The model under review builds one solid part; all positions refer to its coordinate system, in mm. Face numbers are marked on the shaded views. A direction names the side the tool comes from. Round coordinates to 2 decimals unless told otherwise and drop trailing zeros. Loops run counter-clockwise (first coordinate to the right, second up) from the corner with the lowest first, then second, coordinate; pieces in that order, holes last. Notation, with made-up numbers: (-31.5, 20.5) -> (8.5, 20.5) arc R23 cw to (8.5, 44.5) -> close; hole circle Ø10 at (88.25, 5.5). An arc over 180 degrees is marked (long way). Return JSON: item names as keys, results as strings. Group by question number.
```python
from build123d import *

# Parameters (mm, degrees)
F0_W          = 24
F0_H          = 25
F1_DEPTH      = 2
F2_R          = 6.25
F3_DEPTH      = 3
F4_W          = 24
F4_H          = 2
F5_DEPTH      = 7
F5_DEPTH_BACK = 2
F7_START      = 12
F6_W          = 4.5
F6_H          = 5
F7_DEPTH      = 3
F8_START      = -12
F8_DEPTH      = 3
F9_R          = 0.5


with BuildPart() as f1:
    # F0 (on Top) → F1 (new body)
    with BuildSketch(Plane.XY):
        Rectangle(F0_W, F0_H)
    extrude(amount=-F1_DEPTH)

    # F2 (on Top) → F3 (join)
    with BuildSketch(Plane.XY):
        Circle(F2_R)
    extrude(amount=F3_DEPTH)

    # F4 (on Top) → F5 (join, two sides)
    with BuildSketch(Plane.XY) as f5_sk:
        with Locations((0, 13.5)):
            Rectangle(F4_W, F4_H)
        with Locations((0, -13.5)):
            Rectangle(F4_W, F4_H)
    extrude(amount=F5_DEPTH)
    extrude(f5_sk.sketch, amount=-F5_DEPTH_BACK)

    # F6 (on Front) → F7 (cut)
    with BuildSketch(Plane.XZ.offset(F7_START)):
        with Locations((-7, 2.5)):
            Rectangle(F6_W, F6_H)
        with Locations((7, 2.5)):
            Rectangle(F6_W, F6_H)
    extrude(amount=F7_DEPTH, mode=Mode.SUBTRACT)

    # F6 (on Front) → F8 (cut)
    with BuildSketch(Plane.XZ.offset(F8_START)):
        with Locations((-7, 2.5)):
            Rectangle(F6_W, F6_H)
        with Locations((7, 2.5)):
            Rectangle(F6_W, F6_H)
    extrude(amount=-F8_DEPTH, mode=Mode.SUBTRACT)

    # F9
    f9_edges = [f1.edges().sort_by_distance(p)[0] for p in [
        (0, -12.5, 7),
        (0, 12.5, 7),
        (12, 12.5, 3.5),
        (12, -12.5, 3.5),
        (-12, -12.5, 3.5),
        (-12, 12.5, 3.5),
    ]]
    fillet(f9_edges, radius=F9_R)


solid = f1.part
```
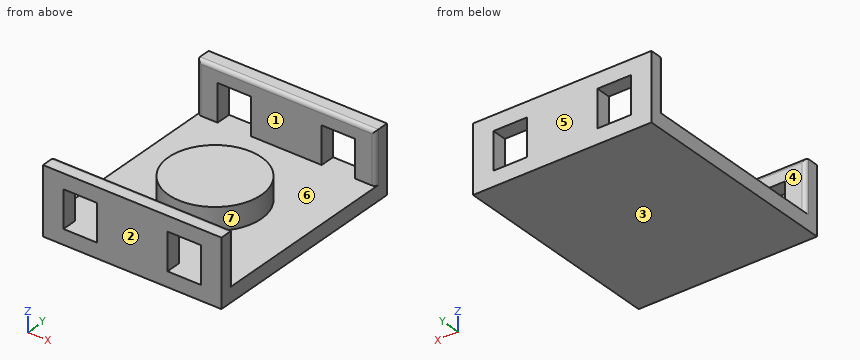
1. We need section D-D, the plane x = 0. Write out the cut boundary in (y, z).
2. We need section C-C, the plane y = 1.75. Write out the cut boundary in (x, z).
3. Tool access review of the marked faces 4, 5, 6 and 7: name each direction out of +Z, -Z, +X, -X, +Y, -Y from which nothing blocks a thin tool from reaching the whole face with its end or side.
4. We need section A-A, the plane z = 4.5. Write out the cut boundary in (x, y), then the cut area to 3 significant figures.
5. Wall thickness on line 1 (Y direction, x = -7.75, z = 6.25); line 2 (Z direction, x = 4, y = -2.25); line 3 (Z direction, x = 9, y = -2.25): over which ranges is each line inside the solid? List them lowest first.
6. We need section B-B, the plane x = 7.75. Write out the cut boundary in (y, z).
7. Draft analysis for pull direction Y (two halves, no side actions). For the marked faces 1, 2 and 3, state which applies: pulls with the +Y half, pulls with the -Y half, needs draft (parallel to the pull), parting line crosses it, or undercut.
8. For P1, Ø6, axis at x = 0.5, y = 2.5, coming from the +Z side; P2, Ø1, axis at y = -5.5, z = 1.5, coming from the +X side, all flat-tipped, find the tip position at first contact; note any pin that passes through.
Check sheet entries:
{
 "1": {"outline": "(-14.5, -2) -> (14.5, -2) -> (14.5, 7) -> (13, 7) arc R0.5 ccw to (12.5, 6.5) -> (12.5, 0) -> (6.25, 0) -> (6.25, 3) -> (-6.25, 3) -> (-6.25, 0) -> (-12.5, 0) -> (-12.5, 6.5) arc R0.5 ccw to (-13, 7) -> (-14.5, 7) -> close"},
 "2": {"outline": "(-12, -2) -> (12, -2) -> (12, 0) -> (6, 0) -> (6, 3) -> (-6, 3) -> (-6, 0) -> (-12, 0) -> close"},
 "3": {"face 4": "+Z, +X, -X", "face 5": "+Z, -Z, +X, -X, +Y", "face 6": "none", "face 7": "+Z"},
 "4": {"outline": "(-12, -14.5) -> (-9.25, -14.5) -> (-9.25, -12.5) -> (-11.5, -12.5) arc R0.5 ccw to (-12, -13) -> close; (-12, 13) arc R0.5 ccw to (-11.5, 12.5) -> (-9.25, 12.5) -> (-9.25, 14.5) -> (-12, 14.5) -> close; (-4.75, -14.5) -> (4.75, -14.5) -> (4.75, -12.5) -> (-4.75, -12.5) -> close; (-4.75, 12.5) -> (4.75, 12.5) -> (4.75, 14.5) -> (-4.75, 14.5) -> close; (9.25, -14.5) -> (12, -14.5) -> (12, -13) arc R0.5 ccw to (11.5, -12.5) -> (9.25, -12.5) -> close; (9.25, 12.5) -> (11.5, 12.5) arc R0.5 ccw to (12, 13) -> (12, 14.5) -> (9.25, 14.5) -> close", "area": "59.8 mm²"},
 "5": {"line 1": "y = -14.5 to -12.5, 12.5 to 14.5", "line 2": "z = -2 to 3", "line 3": "z = -2 to 0"},
 "6": {"outline": "(-14.5, -2) -> (14.5, -2) -> (14.5, 0) -> (-14.5, 0) -> close; (-14.5, 5) -> (-12.5, 5) -> (-12.5, 6.5) arc R0.5 ccw to (-13, 7) -> (-14.5, 7) -> close; (12.5, 5) -> (14.5, 5) -> (14.5, 7) -> (13, 7) arc R0.5 ccw to (12.5, 6.5) -> close"},
 "7": {"face 1": "undercut", "face 2": "pulls with the -Y half", "face 3": "needs draft"},
 "8": {"P1": "stops at z = 3", "P2": "stops at x = 3.75"}
}
